Here's how the part is built. I have some questions about the finished solid (model axes, mm). A direction names the side the tool comes from. Round coordinates to 2 decimals unless told otherwise and drop trailing zeros. Write each loop counter-clockwise with the first axis right and the second up, starting at its lowest first coordinate (ties: lowest second). Pieces come first, ordered by that corner, then holes. Notation, with made-up numbers: (63, 8.25) - (91, 8.25) arc R18 cw to (91, 13.25) - close; hole circle Ø6 at (27, -18.5). An arc over 180 degrees is marked (long way). Use one line per item in the form item = value. Start each with the question number.
1. Which directions (+Z, -Z, +X, -X, +Y, -Y) give clear straight access to the entire face, cutting with the end or side of a thin tool? Please do faces 4 (the flat face through (-284, 7.5, 9)), 5 (the flat face through (284, -7.5, 9)), 6 (the flat face through (293, -15, 9)).
2. I want a section at A-A, the plane z = 3.75. List the corners of the cut face in (x, y) for me, plus the area to 3 significant figures.
3. Will these pins go through, and if not, where does the flat tip stop? pin 1 (4.5 mm diameter, centred on y = -2.5, z = 9, fed in from -X); pin 2 (1.5 mm diameter, centred on y = -2.5, z = 2.5, fed in from +X).
4. We'd pull the mould along Y, two halves only. Please class faces 1 (the flat face through (-4, 0, 0)), 2 (the flat face through (-284, -7.5, 9)), 3 (the flat face through (-4, -22.5, 9)): +Y half, -Y half, draft (parallel to the pull), parting line (faces both ways), or undercut.
5. I want a section at B-B, the plane y = -1.5. List the corners of the cut face in (x, z) for me, plus the area to 3 significant figures.
6. If I drill on line 1 along X through (y, z) = (-2, 8.75), over which ranges is the centre line in solid material (lowest first)?
```python
from build123d import *

# Parameters (mm, degrees)
SKETCH1_W             = 586
SKETCH1_H             = 45
EXTRUDE_357_DEPTH     = 18
CUT_EXTRUDE_572_REACH = 296.413
SKETCH2_W             = 18
SKETCH2_H             = 15


with BuildPart() as part:
    # Sketch1 → Extrude 357 (new body)
    with BuildSketch(Plane.XY):
        Rectangle(SKETCH1_W, SKETCH1_H)
    extrude(amount=EXTRUDE_357_DEPTH)

    # Sketch2 → Cut-Extrude 572 (cut, up to next)
    with BuildSketch(Plane.XY.offset(18), mode=Mode.PRIVATE) as cut_extrude_572_sk1:
        with Locations((-284, 0)):
            Rectangle(SKETCH2_W, SKETCH2_H)
    cut_extrude_572_tool1 = extrude(cut_extrude_572_sk1.sketch, amount=-CUT_EXTRUDE_572_REACH, mode=Mode.PRIVATE) & part.part
    cut_extrude_572 = cut_extrude_572_tool1.solids().sort_by_distance((-284, 0, 18))[0]
    add(cut_extrude_572, mode=Mode.SUBTRACT)

    # Mirror1: Cut-Extrude 572 across plane
    add(cut_extrude_572.mirror(Plane(origin=(0, 0, 0), x_dir=(0, 0, 1), z_dir=(1, 0, 0))), mode=Mode.SUBTRACT)


solid = part.part
```
Model answer:
q1.face_4 = +Z, -Z, -X
q1.face_5 = +Z, -Z, +X
q1.face_6 = +Z, -Z, +X, +Y, -Y
q2.outline = (-293, -22.5) - (293, -22.5) - (293, -7.5) - (275, -7.5) - (275, 7.5) - (293, 7.5) - (293, 22.5) - (-293, 22.5) - (-293, 7.5) - (-275, 7.5) - (-275, -7.5) - (-293, -7.5) - close
q2.area = 25,800 mm2
q3.pin_1 = -275
q3.pin_2 = 275
q4.face_1 = draft
q4.face_2 = undercut
q4.face_3 = -Y half
q5.outline = (-275, 0) - (275, 0) - (275, 18) - (-275, 18) - close
q5.area = 9,900 mm2
q6.line_1 = -275 to 275
